from build123d import *

# Parameters (mm, degrees)
F1_DEPTH = 12.7
F2_R     = 8.7757
F3_DEPTH = 12.7
F4_R     = 4.6736
F5_DEPTH = 12.7


with BuildPart() as f1:
    # F0 (on Front) → F1 (new body, symmetric)
    with BuildSketch(Plane.XZ):
        Polygon((11.991823, 0), (0, 0), (-38.808177, 0), (-38.808177, -17.78), (11.991823, -17.78), align=None)
    extrude(amount=F1_DEPTH, both=True)

    # F2 (on Top) → F3 (cut)
    with BuildSketch(Plane.XY):
        with Locations((-26.108177, 0)):
            Circle(F2_R)
        Circle(F2_R)
    extrude(amount=-F3_DEPTH, mode=Mode.SUBTRACT)

    # F4 (on Right) → F5 (cut, symmetric)
    with BuildSketch(Plane.YZ):
        with Locations((0, -10.830815)):
            Circle(F4_R)
    extrude(amount=F5_DEPTH, both=True, mode=Mode.SUBTRACT)


solid = f1.part
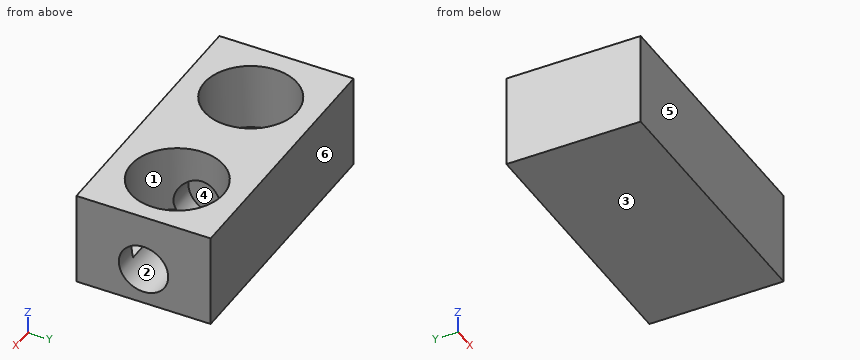
Geometry: final body of the model. Coordinates: model frame, mm. Face numbers are marked on the shaded views. A direction names the side the tool comes from. Coordinates: 2 decimals unless noted, no trailing zeros. Loops run counter-clockwise (first coordinate to the right, second up) from the corner with the lowest first, then second, coordinate; pieces in that order, holes last. Notation, with made-up numbers: (0.5, -37) - (58.5, -37) arc R14 cw to (58.5, -22) - close; hole circle Ø6 at (-37, -4.5). An arc over 180 degrees is marked (long way). One line per question, with ' | ' between items. Start each with the question number.
(1) Ray query, L1, parallel to X at y = 5.5, z = -10.25; L2, parallel to Y at x = 0, z = -6.75; L3, parallel to X at y = 1.5, z = -6. Return the intervals inside material, ascending. Write a range as from..to.
(2) Cut plane C-C on z = -8.75. Output: boundary loops of the cut face in (x, y).
(3) Draft query along Y for the marked faces 4, 5 and 6. Return one class per face: +Y half, -Y half, draft (parallel to the pull), parting line (faces both ways), or undercut.
(4) Reachability of the marked faces 1, 2 and 3 from +Z, -Z, +X, -X, +Y, -Y: full face, straight path, thin tool, end or side. Return the list, or none.
(5) Cut plane D-D on y = -8. Output: boundary loops of the cut face in (x, z).
(6) Cut plane A-A on y = 0. Output: boundary loops of the cut face in (x, z).
(7) First-contact query: pin 1 (3 mm diameter, centred on y = -1.5, z = -10, fed in from +X); pin 2 (5 mm diameter, centred on x = 1, y = 1, fed in from +Z); pin 3 (1.5 mm diameter, centred on x = -25, y = 4, fed in from +Z). Flat tips, straight axial feed; report the tip coordinate or a pass-through.
(8) Cut plane B-B on x = 0. Output: boundary loops of the cut face in (y, z), and give its area (3 significant figures).
Here are the results:
1) L1: -38.81..-32.95, -19.27..-6.84, 6.84..11.99 | L2: -12.7..-8.78, 8.78..12.7 | L3: -38.81..-34.75, -17.46..-8.65, 8.65..11.99
2) outline: (-38.81, -12.7) - (11.99, -12.7) - (11.99, -4.18) - (7.71, -4.18) arc R8.78 cw to (-7.71, -4.18) - (-12.7, -4.18) - (-12.7, 4.18) - (-7.71, 4.18) arc R8.78 cw to (7.71, 4.18) - (11.99, 4.18) - (11.99, 12.7) - (-38.81, 12.7) - close; hole circle Ø17.55 at (-26.11, 0)
3) face 4: undercut | face 5: -Y half | face 6: +Y half
4) face 1: +Z | face 2: +X | face 3: -Z, +X, -X, +Y, -Y
5) outline: (-38.81, -17.78) - (11.99, -17.78) - (11.99, 0) - (3.61, 0) - (3.61, -12.7) - (-3.61, -12.7) - (-3.61, 0) - (-22.5, 0) - (-22.5, -12.7) - (-29.72, -12.7) - (-29.72, 0) - (-38.81, 0) - close
6) outline: (-38.81, -17.78) - (11.99, -17.78) - (11.99, -15.5) - (-12.7, -15.5) - (-12.7, -6.16) - (-8.78, -6.16) - (-8.78, 0) - (-17.33, 0) - (-17.33, -12.7) - (-34.88, -12.7) - (-34.88, 0) - (-38.81, 0) - close; (8.78, -6.16) - (11.99, -6.16) - (11.99, 0) - (8.78, 0) - close
7) pin 1: x = -12.7 | pin 2: z = -13.93 | pin 3: z = -12.7
8) outline: (-12.7, -17.78) - (12.7, -17.78) - (12.7, 0) - (8.78, 0) - (8.78, -12.7) - (4.28, -12.7) arc R4.67 cw to (-4.28, -12.7) - (-8.78, -12.7) - (-8.78, 0) - (-12.7, 0) - close | area: 211 mm²
